Check sheet for the modelled part. Datum: model origin and axes. Units: mm. Round coordinates to 2 decimals unless told otherwise and drop trailing zeros. Write each loop counter-clockwise with the first axis right and the second up, starting at its lowest first coordinate (ties: lowest second). Pieces come first, ordered by that corner, then holes. Notation, with made-up numbers: (84.5, 50) -> (116.5, 50) arc R32 ccw to (116.5, 89) -> close; hole circle Ø5 at (76, 20.25). An arc over 180 degrees is marked (long way). One line per item, written item: value.
Autodesk Inventor part; units mm, degrees
ref_plane "YZ Plane" through (0, 0, 0) normal (1, 0, 0) x (0, 1, 0)
ref_plane "XZ Plane" through (0, 0, 0) normal (0, 1, 0) x (-1, 0, 0)
ref_plane "XY Plane" through (0, 0, 0) normal (0, 0, 1) x (1, 0, 0)
sketch "Sketch1" plane through (0, 0, 0) normal (1, 0, 0) x (0, 1, 0)
  line L0 (0, 0) -> (25.4, 0)
  line L1 (25.4, 0) -> (25.4, -25.4)
  line L2 (25.4, -25.4) -> (0, -25.4)
  line L3 (0, -25.4) -> (0, 0)
  line L4 (3.175, -3.175) -> (22.225, -3.175)
  line L5 (22.225, -3.175) -> (22.225, -22.225)
  line L6 (22.225, -22.225) -> (3.175, -22.225)
  line L7 (3.175, -22.225) -> (3.175, -3.175)
  dimension "d0" = 25.4
  dimension "d1" = 25.4
  dimension "d2" = 19.05
  dimension "d3" = 19.05
  dimension "d4" = 3.175
  dimension "d5" = 3.175
extrude "Extrusion1" add sketch "Sketch1" along normal blind 635
sketch "Sketch2" plane through (0, 0, 0) normal (0, 0, 1) x (1, 0, 0)
  line L0 (0, 0) -> (0, 25.4)
  line L1 (0, 0) -> (635, 0)
  line L2 (635, 25.4) -> (635, 0)
  point P0 (536.575, 12.7)
  point P1 (498.475, 12.7)
  point P2 (136.525, 12.7)
  point P3 (98.425, 12.7)
  dimension "d8" = 98.425
  dimension "d9" = 38.1
  dimension "d10" = 12.7
  dimension "d11" = 12.7
  dimension "d12" = 12.7
  dimension "d13" = 98.425
  dimension "d14" = 38.1
  dimension "d15" = 12.7
hole "Hole1" at (536.575, 12.7, 0) at (498.475, 12.7, 0) at (136.525, 12.7, 0) at (98.425, 12.7, 0) direction (0, 0, -1) diameter 6.35 end through all
sketch "Sketch3" plane through (0, 0, 0) normal (0, 0, 1) x (1, 0, 0)
  line L0 (0, 0) -> (0, 25.4)
  line L1 (0, 0) -> (635, 0)
  line L2 (635, 25.4) -> (635, 0)
  point P0 (12.7, 12.7)
  point P1 (622.3, 12.7)
  dimension "d23" = 12.7
  dimension "d24" = 12.7
  dimension "d25" = 12.7
  dimension "d26" = 12.7
hole "Hole2" at (12.7, 12.7, 0) at (622.3, 12.7, 0) direction (0, 0, -1) diameter 6.35 end through all
sketch "Sketch4" plane through (0, 0, 0) normal (0, 0, 1) x (1, 0, 0)
  line L0 (0, 0) -> (0, 25.4)
  line L1 (0, 0) -> (635, 0)
  line L2 (635, 25.4) -> (635, 0)
  point P0 (76.2, 12.7)
  point P1 (228.6, 12.7)
  point P2 (406.4, 12.7)
  point P3 (558.8, 12.7)
  dimension "d34" = 12.7
  dimension "d35" = 12.7
  dimension "d36" = 12.7
  dimension "d37" = 12.7
  dimension "d38" = 76.2
  dimension "d39" = 228.6
  dimension "d40" = 228.6
  dimension "d41" = 76.2
hole "Hole3" at (76.2, 12.7, 0) at (228.6, 12.7, 0) at (406.4, 12.7, 0) at (558.8, 12.7, 0) direction (0, 0, -1) diameter 4.7625 end through all
sketch "Sketch6" plane through (0, 0, -25.4) normal (0, 0, -1) x (-1, 0, 0)
  circle A0 centre (-136.525, 12.7) radius 3.175
  circle A1 centre (-498.475, 12.7) radius 3.175
  line L0 (0, 0) -> (-635, 0)
  circle A2 centre (-492.125, 12.7) radius 3.175
  circle A3 centre (-142.875, 12.7) radius 3.175
  dimension "d61" = 6.35
  dimension "d62" = 6.35
  dimension "d63" = 6.35
  dimension "d64" = 12.7
  dimension "d65" = 6.35
  dimension "d66" = 12.7
extrude "Extrusion2" cut sketch "Sketch6" against normal blind 25.4 contours A3 | A2
sketch "Sketch7" plane through (0, 25.4, 0) normal (0, 1, 0) x (1, 0, 0)
  line L0 (635, 25.4) -> (635, 0)
  line L1 (0, 25.4) -> (635, 25.4)
  point P0 (504.825, 12.7)
  point P1 (130.175, 12.7)
  dimension "d69" = 12.7
  dimension "d70" = 130.175
  dimension "d71" = 12.7
  dimension "d81" = 374.65
hole "Hole5" at (504.825, 25.4, -12.7) at (130.175, 25.4, -12.7) direction (0, -1, 0) diameter 4.7625 depth 25.4 tip angle 118
properties part number "1x1 horizontal" material "Aluminum 6061"
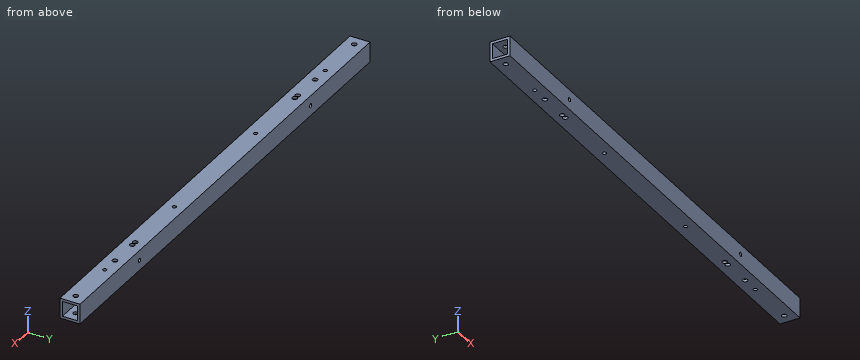
Item 1: Thickness scan on line 1 (X direction, y = 2, z = -12.7); line 2 (Y direction, x = 48, z = -8.25) (3 decimals); line 3 (Z direction, x = 315, y = 7.75) (3 decimals). Record the ranges inside material, lowest first.
Answer:
line 1: x = 0 to 127.79, 132.56 to 502.44, 507.21 to 635
line 2: y = 0 to 3.175, 22.225 to 25.4
line 3: z = -25.4 to -22.225, -3.175 to 0
Item 2: Sectioned sample at A-A on x = 293. Enter the section's corners in (y, z) (3 decimals).
Answer:
outline: (0, -25.4) -> (25.4, -25.4) -> (25.4, 0) -> (0, 0) -> close; hole (3.175, -22.225) -> (22.225, -22.225) -> (22.225, -3.175) -> (3.175, -3.175) -> close
Item 3: Depth check by flat-ended pin: P1, Ø5.5, axis at x = 142.875, y = 12.7, coming from the -Z side; P2, Ø12, axis at y = 3.5, z = -16, coming from the +X side. Enter the tip coordinate at first touch or a pass-through.
Answer:
P1: passes through
P2: stops at x = 635
